The drawing under review shows one solid part. Ordinate dimensions are in mm from its lowest x, y, z. A direction names the side the tool comes from. Give positions to 0.01 mm unless a question says otherwise; leave off trailing zeros. Write each loop counter-clockwise with the first axis right and the second up, starting at its lowest first coordinate (ties: lowest second). Pieces come first, ordered by that corner, then holes. Notation, with made-up numbers: (57.5, 37) -> (62.5, 37) arc R24 cw to (62.5, 60) -> close; hole circle Ø4 at (48.25, 61.25). An arc over 180 degrees is marked (long way). Answer as a JSON object with one key per item and string values.
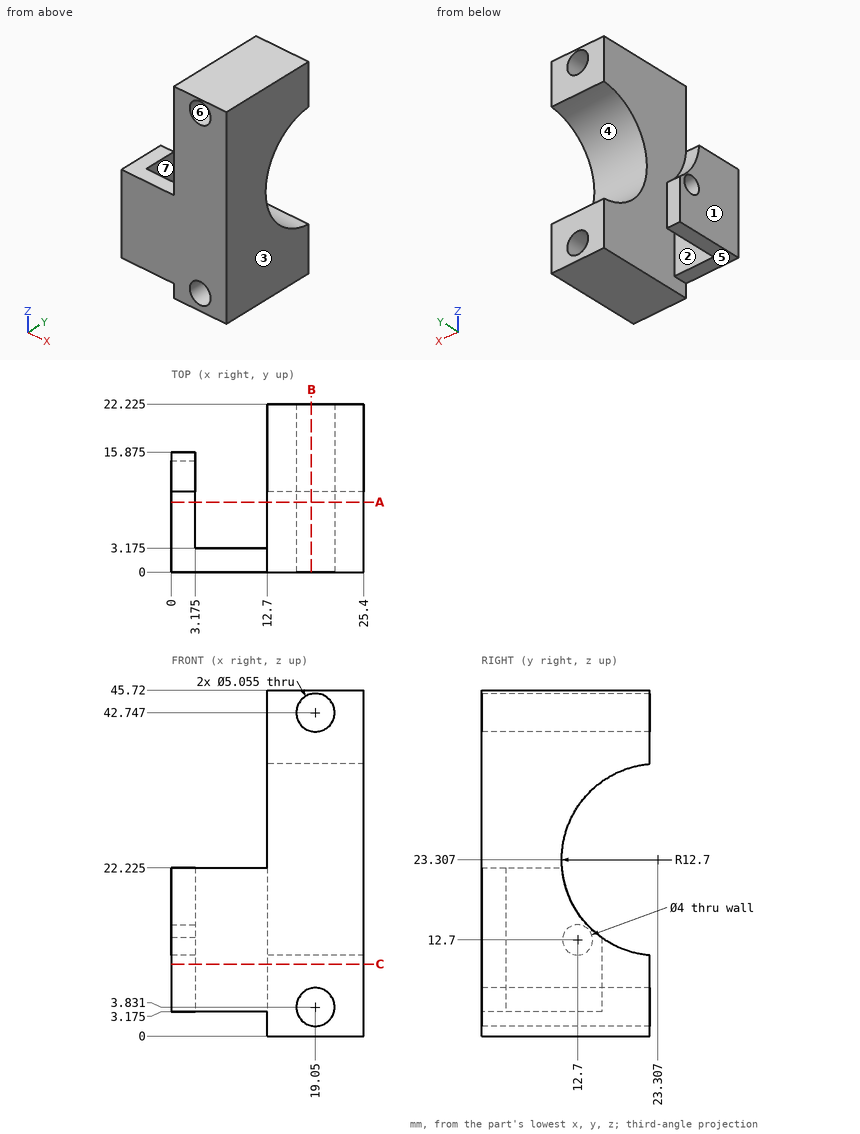
(1) We need section A-A, the plane y = 9.25. Give the number of separate pieces and of enclosed holes in the cut face, then the cut area to 3 significant figures.
Here are the results:
{"separate pieces": "2", "enclosed holes": "2", "area": "601 mm²"}
(2) Clearance check with flat-ended pins moving along their axes: pin 1 (10 mm diameter, centred on x = 3, y = 5.5, fed in from -Z) (3 decimals); pin 2 (4 mm diameter, centred on x = 19.05, z = 3.83, fed in from -Y); pin 3 (5.5 mm diameter, centred on x = 3.5, y = 4.5, fed in from +Z) (3 decimals); pin 4 (5 mm diameter, centred on x = 3, z = 6, fed in from +Y) (3 decimals). State where each tip first meets the part, or that it passes through.
Here are the results:
{"pin 1": "stops at z = 3.175", "pin 2": "passes through", "pin 3": "stops at z = 22.225", "pin 4": "stops at y = 15.875"}
(3) For line 1 along X through (y, z) = (15, 13) (1 decimal); line 2 along Z through (x, y) = (18.5, 7.5) (1 decimal); line 3 along Z through (x, y) = (19.05, 12.5) (1 decimal), list the stretches that pass through material, from the lowest coordinate up.
Here are the results:
{"line 1": "x = 0 to 3.2, 12.7 to 25.4", "line 2": "z = 0 to 1.4, 6.3 to 40.3, 45.2 to 45.7", "line 3": "z = 0 to 1.3, 6.4 to 16.6, 30 to 40.2, 45.3 to 45.7"}
(4) The part is to be moulded in two halves that separate along X. For the marked faces 1, 2, 3 and 4, say which applies: +X half, -X half, draft (parallel to the pull), parting line (faces both ways), or undercut.
Here are the results:
{"face 1": "-X half", "face 2": "undercut", "face 3": "+X half", "face 4": "draft"}
(5) For the marked faces 5, 6 and 7, list the 3-axis set-ups (+Z, -Z, +X, -X, +Y, -Y) from which the entire face can be reached by the end or side of a thin tool; tool diameter is ignored.
Here are the results:
{"face 5": "-Z, -X, +Y, -Y", "face 6": "+Y, -Y", "face 7": "+Z, -Z, +Y"}
(6) We need section B-B, the plane x = 18.5. State the section outline as (y, z) points (1 decimal), then the cut area to 3 significant figures.
Here are the results:
{"outline": "(0, 0) -> (22.2, 0) -> (22.2, 1.4) -> (0, 1.4) -> close; (0, 6.3) -> (22.2, 6.3) -> (22.2, 10.7) arc R12.7 cw to (22.2, 36) -> (22.2, 40.3) -> (0, 40.3) -> close; (0, 45.2) -> (22.2, 45.2) -> (22.2, 45.7) -> (0, 45.7) -> close", "area": "571 mm²"}
(7) We need section C-C, the plane z = 9.5. State the section outline as (x, y) points (1 decimal), then the cut area to 3 significant figures.
Here are the results:
{"outline": "(0, 0) -> (25.4, 0) -> (25.4, 22.2) -> (12.7, 22.2) -> (12.7, 3.2) -> (3.2, 3.2) -> (3.2, 15.9) -> (0, 15.9) -> close", "area": "363 mm²"}
